```python
from build123d import *

# Parameters (mm, degrees)
SKETCH005_R             = 1.65
PAD001_DEPTH            = 8.5
POCKET001_DEPTH         = 5.5
SKETCH008_R             = 0.8
SKETCH011_W             = 25
SKETCH011_H             = 72
POCKET003_DEPTH         = 6
SKETCH012_R             = 1.05
PAD003_DEPTH            = 10
BODY001_PLACEMENT_ANGLE = 180


with BuildPart() as part:
    # Sketch005 → Pad001 (new body)
    with BuildSketch(Plane.XY):
        with BuildLine():
            Line((-47.5, 53.5), (-47.5, -53.5))
            ThreePointArc((-47.5, -53.5), (-46.328427, -56.328427), (-43.5, -57.5))
            Line((-43.5, -57.5), (43.5, -57.5))
            ThreePointArc((43.5, -57.5), (46.328427, -56.328427), (47.5, -53.5))
            Line((47.5, 53.5), (47.5, -53.5))
            ThreePointArc((47.5, 53.5), (46.328427, 56.328427), (43.5, 57.5))
            Line((-43.5, 57.5), (43.5, 57.5))
            ThreePointArc((-43.5, 57.5), (-46.328427, 56.328427), (-47.5, 53.5))
        make_face()
        with Locations((-43.5, 53.5)):
            Circle(SKETCH005_R, mode=Mode.SUBTRACT)
        with Locations((43.5, -53.5)):
            Circle(SKETCH005_R, mode=Mode.SUBTRACT)
        with Locations((-43.5, -53.5)):
            Circle(SKETCH005_R, mode=Mode.SUBTRACT)
        with Locations((43.5, 53.5)):
            Circle(SKETCH005_R, mode=Mode.SUBTRACT)
    extrude(amount=PAD001_DEPTH)

    # Sketch006 (on Face14 of Pad001) → Pocket001 (cut)
    with BuildSketch(Plane.XY.offset(8.5)):
        with BuildLine():
            ThreePointArc((-40.5, 46.5), (-37.671573, 47.671573), (-36.5, 50.5))
            Line((-36.5, 50.5), (-36.5, 54.5))
            Line((-36.5, 54.5), (36.5, 54.5))
            Line((36.5, 50.5), (36.5, 54.5))
            ThreePointArc((36.5, 50.5), (37.671573, 47.671573), (40.5, 46.5))
            Line((40.5, 46.5), (44.5, 46.5))
            Line((44.5, -46.5), (44.5, 46.5))
            Line((40.5, -46.5), (44.5, -46.5))
            ThreePointArc((40.5, -46.5), (37.671573, -47.671573), (36.5, -50.5))
            Line((36.5, -54.5), (36.5, -50.5))
            Line((-36.5, -54.5), (36.5, -54.5))
            Line((-36.5, -50.5), (-36.5, -54.5))
            ThreePointArc((-36.5, -50.5), (-37.671573, -47.671573), (-40.5, -46.5))
            Line((-40.5, -46.5), (-44.5, -46.5))
            Line((-44.5, 46.5), (-44.5, -46.5))
            Line((-40.5, 46.5), (-44.5, 46.5))
        make_face()
    extrude(amount=-POCKET001_DEPTH, mode=Mode.SUBTRACT)

    # SubtractivePipe001: sweep along a path in Sketch007
    with BuildLine(Plane.XY) as subtractivepipe001_path:
        ThreePointArc((42.585786, -49.757359), (40.792635, -50.792635), (39.757359, -52.585786))
        Line((39.757359, -52.585786), (39.239721, -54.517638))
        ThreePointArc((39.239721, -54.517638), (38.525392, -55.586707), (37.30787, -56))
        Line((37.30787, -56), (-37.30787, -56))
        ThreePointArc((-37.30787, -56), (-38.525392, -55.586707), (-39.239721, -54.517638))
        Line((-39.239721, -54.517638), (-39.757359, -52.585786))
        ThreePointArc((-39.757359, -52.585786), (-40.792635, -50.792635), (-42.585786, -49.757359))
        Line((-42.585786, -49.757359), (-44.517638, -49.239721))
        ThreePointArc((-44.517638, -49.239721), (-45.586707, -48.525392), (-46, -47.30787))
        Line((-46, -47.30787), (-46, 47.30787))
        ThreePointArc((-46, 47.30787), (-45.586707, 48.525392), (-44.517638, 49.239721))
        Line((-44.517638, 49.239721), (-42.585786, 49.757359))
        ThreePointArc((-42.585786, 49.757359), (-40.792635, 50.792635), (-39.757359, 52.585786))
        Line((-39.757359, 52.585786), (-39.239721, 54.517638))
        ThreePointArc((-39.239721, 54.517638), (-38.525392, 55.586707), (-37.30787, 56))
        Line((-37.30787, 56), (37.30787, 56))
        ThreePointArc((37.30787, 56), (38.525392, 55.586707), (39.239721, 54.517638))
        Line((39.239721, 54.517638), (39.757359, 52.585786))
        ThreePointArc((39.757359, 52.585786), (40.792635, 50.792635), (42.585786, 49.757359))
        Line((42.585786, 49.757359), (44.517638, 49.239721))
        ThreePointArc((44.517638, 49.239721), (45.586707, 48.525392), (46, 47.30787))
        Line((46, 47.30787), (46, -47.30787))
        ThreePointArc((46, -47.30787), (45.586707, -48.525392), (44.517638, -49.239721))
        Line((44.517638, -49.239721), (42.585786, -49.757359))
    # Sketch008 → SubtractivePipe001 (sweep, cut)
    with BuildSketch(Plane.XZ):
        with Locations((46, 8.5)):
            Circle(SKETCH008_R)
    sweep(path=subtractivepipe001_path.line, mode=Mode.SUBTRACT)

    # Sketch011 (on Face56 of SubtractivePipe001) → Pocket003 (cut)
    with BuildSketch(Plane.XY.offset(3)):
        with Locations((22.5, 0)):
            Rectangle(SKETCH011_W, SKETCH011_H)
    extrude(amount=-POCKET003_DEPTH, mode=Mode.SUBTRACT)

    # Sketch012 (on Face43 of Pocket003) → Pad003 (join)
    with BuildSketch(Plane.XY.offset(3)):
        with BuildLine():
            Line((5.5, 40), (39.5, 40))
            ThreePointArc((40.5, 39), (40.207107, 39.707107), (39.5, 40))
            Line((40.5, 39), (40.5, 36.5))
            ThreePointArc((36.317588, 34.767588), (38.987574, 34.236495), (40.5, 36.5))
            Line((36.317588, 34.767588), (35, 36.085177))
            Line((10, 36.085177), (35, 36.085177))
            Line((8.682412, 34.767588), (10, 36.085177))
            ThreePointArc((4.5, 36.5), (6.012426, 34.236495), (8.682412, 34.767588))
            Line((4.5, 39), (4.5, 36.5))
            ThreePointArc((5.5, 40), (4.792893, 39.707107), (4.5, 39))
        make_face()
        with Locations((38, 37.5)):
            Circle(SKETCH012_R, mode=Mode.SUBTRACT)
        with Locations((7, 37.5)):
            Circle(SKETCH012_R, mode=Mode.SUBTRACT)
        with BuildLine():
            Line((5.5, -40), (39.5, -40))
            ThreePointArc((39.5, -40), (40.207107, -39.707107), (40.5, -39))
            Line((40.5, -39), (40.5, -36.5))
            ThreePointArc((40.5, -36.5), (38.987574, -34.236495), (36.317588, -34.767588))
            Line((35, -36.085177), (36.317588, -34.767588))
            Line((10, -36.085177), (35, -36.085177))
            Line((8.682412, -34.767588), (10, -36.085177))
            ThreePointArc((8.682412, -34.767588), (6.012426, -34.236495), (4.5, -36.5))
            Line((4.5, -39), (4.5, -36.5))
            ThreePointArc((4.5, -39), (4.792893, -39.707107), (5.5, -40))
        make_face()
        with Locations((7, -37.5)):
            Circle(SKETCH012_R, mode=Mode.SUBTRACT)
        with Locations((38, -37.5)):
            Circle(SKETCH012_R, mode=Mode.SUBTRACT)
    extrude(amount=PAD003_DEPTH)


with BuildPart() as part_1:
    # Body001 placement: moved
    add(part.part.moved(Location((0, 0, 45.5))).rotate(Axis((0, 0, 45.5), (1, 0, 0)), BODY001_PLACEMENT_ANGLE))


solid = part_1.part
```
Part model, mm, in its own coordinate system. A direction names the side the tool comes from. Round coordinates to 2 decimals unless told otherwise and drop trailing zeros. Loops run counter-clockwise (first coordinate to the right, second up) from the corner with the lowest first, then second, coordinate; pieces in that order, holes last. Notation, with made-up numbers: (4.5, 50) -> (8.5, 50) arc R16 ccw to (8.5, 73) -> close; hole circle Ø2 at (61.25, 8). An arc over 180 degrees is marked (long way). Use one line per item in the form item = value. Start each with the question number.
Item 1: Two-plate mould, pull along X, no slides. Class faces 1 (the cylindrical face through (39.02, 34.25, 37.57)), 2 (the cylindrical face through (-46.359, 56.297, 41.309)), 3 (the cylindrical face through (46.297, 56.359, 41.309)), 4 (the flat face through (23, -38, 32.5)): released by +X, released by -X, zero draft, split by the parting line, or undercut.
Item 2: Band-saw the part on A-A (z = 35.75). List the corners of the cut face in (x, y), plus the area to 3 significant figures.
Item 3: Drop flat-ended pins along their axis: pin 1 Ø0.8 at (y, z) = (38.5, 35) entering from +X; pin 2 Ø8 at (x, y) = (17, -31) entering from +Z; pin 3 Ø5.5 at (x, y) = (-43.5, -53.5) entering from -Z; pin 4 Ø3 at (x, z) = (17.5, 35) entering from -Y. Give the stop position or say it passes through.
Item 4: Drill centre lines: line 1 along X through (y, z) = (53.5, 42.25); line 2 along Y through (x, z) = (-43.5, 41); line 3 along X through (y, z) = (-37.5, 36.75). Where is each one in solid material? Low to high.
Item 5: Band-saw the part on B-B (z = 41.25). Give the number of separate pieces and of enclosed holes in the cut face, plus the area to 3 significant figures.
Item 6: Tool access for faces 5 (the flat face through (22, 40, 38)), 6 (the flat face through (-1, 57.5, 41)), 7 (the flat face through (35, 1, 44)): list every direction of +Z, -Z, +X, -X, +Y, -Y with a clear straight run to the whole face (end or side of a thin tool).
Data:
q1.face_1 = undercut
q1.face_2 = released by -X
q1.face_3 = released by +X
q1.face_4 = zero draft
q2.outline = (4.5, -39) arc R1 ccw to (5.5, -40) -> (39.5, -40) arc R1 ccw to (40.5, -39) -> (40.5, -36.5) arc R2.45 ccw to (36.32, -34.77) -> (35, -36.09) -> (10, -36.09) -> (8.68, -34.77) arc R2.45 ccw to (4.5, -36.5) -> close; (4.5, 36.5) arc R2.45 ccw to (8.68, 34.77) -> (10, 36.09) -> (35, 36.09) -> (36.32, 34.77) arc R2.45 ccw to (40.5, 36.5) -> (40.5, 39) arc R1 ccw to (39.5, 40) -> (5.5, 40) arc R1 ccw to (4.5, 39) -> close; hole circle Ø2.1 at (7, -37.5); hole circle Ø2.1 at (7, 37.5); hole circle Ø2.1 at (38, -37.5); hole circle Ø2.1 at (38, 37.5)
q2.area = 298 mm^2
q3.pin_1 = 40.5
q3.pin_2 = through
q3.pin_3 = 37
q3.pin_4 = -40
q4.line_1 = -47.5 to -45.15, -41.85 to -36.5, 36.5 to 41.85, 45.15 to 47.5
q4.line_2 = -57.5 to -55.15, -51.85 to -46.5, 46.5 to 51.85, 55.15 to 57.5
q4.line_3 = 4.5 to 5.95, 8.05 to 36.95, 39.05 to 40.5
q5.separate_pieces = 3
q5.enclosed_holes = 9
q5.area = 1,720 mm^2
q6.face_5 = -Z
q6.face_6 = +Z, -Z, +X, -X, +Y
q6.face_7 = +Z, -Z
